Design review of the part shown in the three views and the two pictorial views. Dimensions are in mm from the part's minimum x, y and z. Coordinates: 2 decimals unless noted, no trailing zeros. Write each loop counter-clockwise with the first axis right and the second up, starting at its lowest first coordinate (ties: lowest second). Pieces come first, ordered by that corner, then holes.
Q1. Take a section at A-A, the plane y = 100. Write out the cut boundary in (x, z).
Q2. For L1, parallel to Z at x = 15.25, y = 100; L2, parallel to Y at x = 5.5, z = 43; L3, parallel to Z at x = 3.75, y = 107, list the stretches that pass through material, from the lowest coordinate up.
Q3. The part is to be moulded in two halves that separate along Z. For the marked faces 1, 2 and 3, say which applies: released by +Z, released by -Z, zero draft, split by the parting line, or undercut.
Q4. Take a section at B-B, the plane z = 100. Write out the cut boundary in (x, y).
Q5. For pin 1 Ø10 at (x, y) = (5, 64.5) entering from +Z; pin 2 Ø1 at (x, y) = (14, 34.5) entering from +Z; pin 3 Ø6 at (x, z) = (8.5, 103) entering from +Y, all flat-tipped, find the tip position at first contact; note any pin that passes through.
Q6. Take a section at C-C, the plane x = 14. Write out the cut boundary in (y, z), plus the area to 3 significant figures.
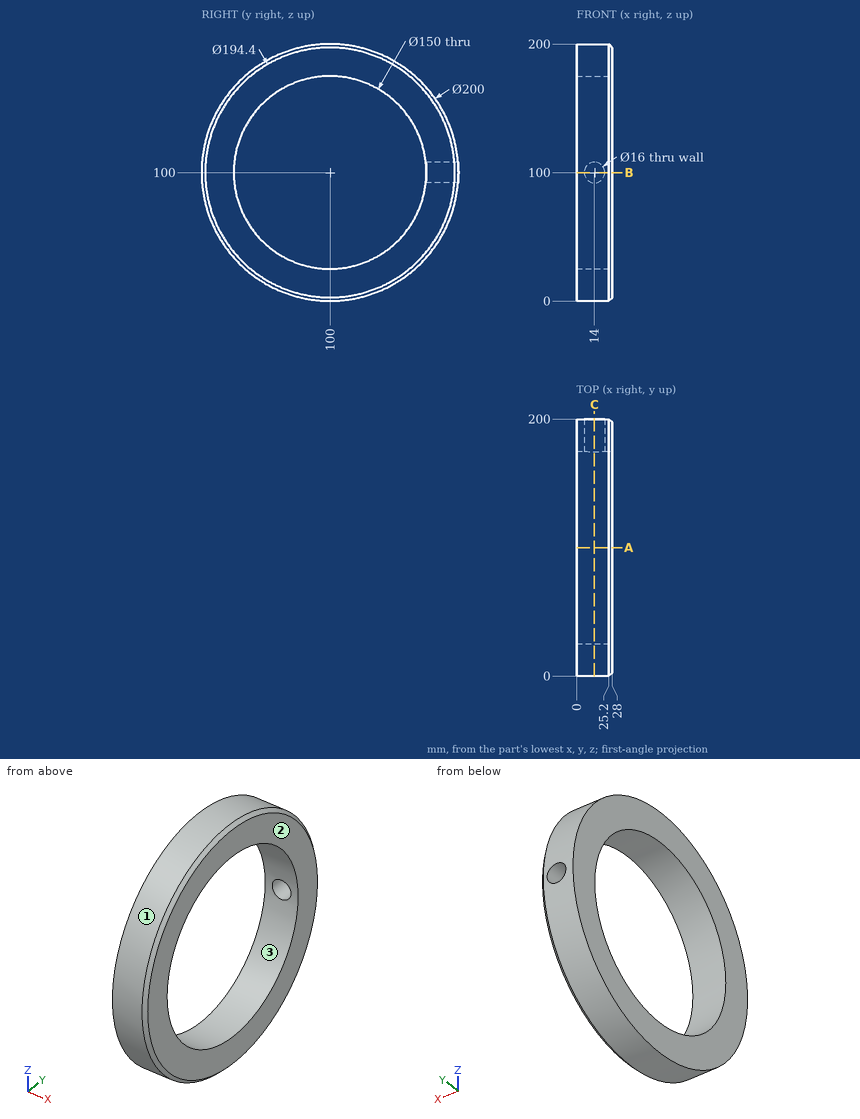
Responses:
1. outline: (0, 0) - (25.2, 0) - (28, 2.8) - (28, 25) - (0, 25) - close; (0, 175) - (28, 175) - (28, 197.2) - (25.2, 200) - (0, 200) - close
2. L1: z = 0 to 25, 175 to 200
2. L2: y = 17.84 to 51.26, 148.74 to 182.16
2. L3: z = 0.25 to 25.33, 174.67 to 199.75
3. face 1: split by the parting line
3. face 2: zero draft
3. face 3: undercut
4. outline: (0, 0) - (25.2, 0) - (28, 2.8) - (28, 25) - (0, 25) - close; (0, 175) - (6, 175) - (6, 200) - (0, 200) - close; (22, 175) - (28, 175) - (28, 197.2) - (25.2, 200) - (22, 200) - close
5. pin 1: stops at z = 195.24
5. pin 2: stops at z = 175.99
5. pin 3: stops at y = 199.99
6. outline: (174.57, 92) arc R75 cw (long way) to (174.57, 108) - (199.68, 108) arc R100 ccw (long way) to (199.68, 92) - close
6. area: 13,300 mm2
